Here's how the part is built. I have some questions about the finished solid (model axes, mm). A direction names the side the tool comes from. Give positions to 0.01 mm unless a question says otherwise; leave off trailing zeros. Write each loop counter-clockwise with the first axis right and the second up, starting at its lowest first coordinate (ties: lowest second). Pieces come first, ordered by that corner, then holes. Notation, with made-up numbers: (-10.75, -8) - (18.25, -8) arc R20 ccw to (18.25, 26) - close; hole circle Ø5 at (-30, -0.75). An arc over 180 degrees is marked (long way). Write each question's results on one line, items separated by ' | '. Start each with the question number.
Item 1: Which directions (+Z, -Z, +X, -X, +Y, -Y) give clear straight access to the entire face, cutting with the end or side of a thin tool? Please do faces 1 (the flat face through (32, 15, -68)), 2 (the flat face through (32, 46, 20)).
Item 2: Will these pins go through, and if not, where does the flat tip stop? P1, Ø8, axis at x = 50, y = 41, coming from the -Z side; P2, Ø19.5, axis at x = 44, z = -65.5, coming from the +Y side.
Item 3: Suppose I cut it at B-B on x = 27. List the corners of the cut face in (y, z) for me.
Item 4: Suppose I cut it at A-A on z = 5.5. List the corners of the cut face in (x, y) for me.
Item 5: Suppose I cut it at C-C on y = 40. List the corners of the cut face in (x, z) for me.
Item 6: Suppose I cut it at D-D on x = 47.5. List the corners of the cut face in (y, z) for me, then the cut area to 3 significant figures.
Item 7: Please list where these lines run through material, in increasing order: line 1 along Y through (x, z) = (16.5, -8.5); line 2 along Z through (x, y) = (41, 17); line 3 along Y through (x, z) = (44, 12.5).
Autodesk Inventor part; units mm, degrees
ref_plane "YZ Plane" through (0, 0, 0) normal (1, 0, 0) x (0, 1, 0)
ref_plane "XZ Plane" through (0, 0, 0) normal (0, 1, 0) x (-1, 0, 0)
ref_plane "XY Plane" through (0, 0, 0) normal (0, 0, 1) x (1, 0, 0)
sketch "Sketch1" plane through (0, 0, 0) normal (0, 0, 1) x (1, 0, 0)
  line L0 (0, 0) -> (65, 0)
  line L1 (65, 0) -> (65, 90)
  line L2 (65, 90) -> (0, 90)
  line L3 (0, 90) -> (0, 0)
  dimension "d0" = 65
  dimension "d1" = 90
extrude "Extrusion1" add sketch "Sketch1" along normal blind 20
fillet "Fillet1" radius 25 1 edges at (65, 90, 10)
sketch "Sketch2" plane through (0, 0, 0) normal (0, 0, -1) x (-1, 0, 0)
  point P0 (0, 0)
sketch "Sketch3" plane through (65, 0, 20) normal (1, 0, 0) x (0, 0, -1)
  point P0 (20, 0)
sketch "Sketch4" plane through (0, 0, 0) normal (0, 0, -1) x (-1, 0, 0)
  point P0 (0, 0)
sketch "Sketch5" plane through (0, 0, 0) normal (0, -1, 0) x (1, 0, 0)
  line L0 (40, 0) -> (0, 0)
  line L1 (0, 0) -> (65, 0)
  line L2 (65, 0) -> (65, -137)
  line L3 (65, -137) -> (0, -137)
  line L4 (0, -137) -> (0, 0)
  dimension "d5" = 65
  dimension "d6" = 137
extrude "Extrusion2" add sketch "Sketch5" against normal blind 15
sketch "Sketch6" plane through (65, 0, -137) normal (0, 0, -1) x (-1, 0, 0)
  line L0 (65, 0) -> (0, 0)
  line L1 (65, 0) -> (78, 0)
  line L2 (78, 0) -> (78, 17)
  line L3 (78, 17) -> (65, 0)
  dimension "d9" = 13
  dimension "d10" = 17
sketch "Sketch7" plane through (65, 0, -137) normal (0, 0, -1) x (-1, 0, 0)
  point P0 (65, 0)
properties part number "YETTOCOMPLETE"
Checked values:
1) face 1: -Z, +X, -X, +Y | face 2: +Z, +X, -X, +Y, -Y
2) P1: stops at z = 0 | P2: stops at y = 15
3) outline: (0, -137) - (15, -137) - (15, 0) - (90, 0) - (90, 20) - (0, 20) - close
4) outline: (0, 0) - (65, 0) - (65, 65) arc R25 ccw to (40, 90) - (0, 90) - close
5) outline: (0, 0) - (65, 0) - (65, 20) - (0, 20) - close
6) outline: (0, -137) - (15, -137) - (15, 0) - (88.85, 0) - (88.85, 20) - (0, 20) - close | area: 3,830 mm^2
7) line 1: y = 0 to 15 | line 2: z = 0 to 20 | line 3: y = 0 to 89.68
